Autodesk Inventor part; units mm, degrees
ref_plane "YZ Plane" through (0, 0, 0) normal (1, 0, 0) x (0, 1, 0)
ref_plane "XZ Plane" through (0, 0, 0) normal (0, 1, 0) x (-1, 0, 0)
ref_plane "XY Plane" through (0, 0, 0) normal (0, 0, 1) x (1, 0, 0)
sketch "Sketch1" plane through (0, 0, 0) normal (0, 0, 1) x (1, 0, 0)
  line L0 (0, 0) -> (30, 0)
  line L1 (30, 0) -> (30, 3)
  line L2 (30, 3) -> (3, 3)
  line L3 (3, 3) -> (3, 30)
  line L4 (3, 30) -> (0, 30)
  line L5 (0, 30) -> (0, 0)
  dimension "d0" = 3
  dimension "d1" = 3
  dimension "d2" = 30
  dimension "d3" = 30
extrude "Extrusion1" add sketch "Sketch1" along normal blind 1800
sketch "Sketch2" plane through (3, 3, 1800) normal (0, 1, 0) x (1, 0, 0)
  line L0 (0, 1800) -> (0, 0)
  line L1 (27, 0) -> (0, 0)
  point P0 (-3, 1800)
  point P1 (15, 15)
  point P2 (15, 465)
  point P3 (15, 915)
  point P4 (15, 1365)
  dimension "d6" = 15
  dimension "d7" = 15
  dimension "d8" = 27
  dimension "d9" = 15
  dimension "d10" = 450
  dimension "d11" = 450
  dimension "d12" = 15
  dimension "d13" = 450
  dimension "d14" = 15
hole "Hole1" at (18, 3, 1785) at (18, 3, 1335) at (18, 3, 885) at (18, 3, 435) direction (0, -1, 0) diameter 3.81 end through all
sketch "Sketch3" plane through (3, 30, 1800) normal (1, 0, 0) x (0, 0, -1)
  line L0 (0, -27) -> (0, 0)
  line L1 (1800, -27) -> (0, -27)
  point P0 (1800, -30)
  point P1 (15, -12)
  point P2 (465, -12)
  point P3 (915, -12)
  point P4 (1365, -12)
  dimension "d22" = 15
  dimension "d23" = 15
  dimension "d24" = 15
  dimension "d25" = 450
  dimension "d26" = 450
  dimension "d27" = 15
  dimension "d28" = 450
  dimension "d29" = 15
hole "Hole2" at (3, 18, 1785) at (3, 18, 1335) at (3, 18, 885) at (3, 18, 435) direction (-1, 0, 0) diameter 3.81 end through all
equation "\"d0\" = Thickness"
equation "\"d1\" = Thickness"
equation "\"d2\" = Width"
equation "\"d3\" = Width"
equation "\"d4\" = Height"
equation "\"Width\" = 30"
equation "\"Thickness\" = 3"
equation "\"Height\" = 1800"
equation "\"HoleDistance\" = 15"
properties part number "corner180"
The model under review builds one solid part; all positions refer to its coordinate system, in mm. Round coordinates to 2 decimals unless told otherwise and drop trailing zeros. Loops run counter-clockwise (first coordinate to the right, second up) from the corner with the lowest first, then second, coordinate; pieces in that order, holes last.
Item 1: Take a section at B-B (x = 11.5). Write out the cut boundary in (y, z).
Determined:
outline: (0, 0) - (3, 0) - (3, 1800) - (0, 1800) - close
Item 2: For line 1 (Z direction, x = 1.6, y = 18) (3 decimals); line 2 (X direction, y = 1.15, z = 885) (3 decimals); line 3 (Y direction, x = 17.5, z = 277), list the stretches that pass through material, from the lowest coordinate up.
Determined:
line 1: z = 0 to 433.095, 436.905 to 883.095, 886.905 to 1333.095, 1336.905 to 1783.095, 1786.905 to 1800
line 2: x = 0 to 16.095, 19.905 to 30
line 3: y = 0 to 3
Item 3: Take a section at A-A (z = 384). Write out the cut boundary in (x, y), then the cut area to 3 significant figures.
Determined:
outline: (0, 0) - (30, 0) - (30, 3) - (3, 3) - (3, 30) - (0, 30) - close
area: 171 mm2
Item 4: Clearance check with flat-ended pins moving along their axes: pin 1 Ø5 at (y, z) = (18, 1785) entering from +X; pin 2 Ø3.5 at (x, z) = (18, 435) entering from -Y; pin 3 Ø8 at (x, z) = (14.5, 759.5) entering from +Y. State where each tip first meets the part, or that it passes through.
Determined:
pin 1: stops at x = 3
pin 2: passes through
pin 3: stops at y = 3
